from build123d import *

# Parameters (mm, degrees)
SKETCH1_W           = 200
SKETCH1_H           = 97
BOSS_EXTRUDE1_DEPTH = 20.75
SKETCH2_W           = 15
SKETCH2_H           = 96
CUT_EXTRUDE1_DEPTH  = 34
SKETCH3_W           = 6.3
SKETCH3_H           = 96
CUT_EXTRUDE2_DEPTH  = 40.5
SKETCH4_R           = 1.65
CUT_EXTRUDE3_DEPTH  = 2
SKETCH5_R           = 1.65
CUT_EXTRUDE4_DEPTH  = 42.5


with BuildPart() as part:
    # Sketch1 → Boss-Extrude1 (new body, symmetric)
    with BuildSketch(Plane(origin=(0, 0, 0), x_dir=(1, 0, 0), z_dir=(0, 1, 0))):
        Rectangle(SKETCH1_W, SKETCH1_H)
    extrude(amount=BOSS_EXTRUDE1_DEPTH, both=True)

    # Sketch2 → Cut-Extrude1 (cut)
    with BuildSketch(Plane(origin=(0, 20.75, 0), x_dir=(1, 0, 0), z_dir=(0, 1, 0))):
        with Locations((92.5, -0.5)):
            Rectangle(SKETCH2_W, SKETCH2_H)
    extrude(amount=-CUT_EXTRUDE1_DEPTH, mode=Mode.SUBTRACT)

    # Sketch3 → Cut-Extrude2 (cut)
    with BuildSketch(Plane(origin=(0, 20.75, 0), x_dir=(1, 0, 0), z_dir=(0, 1, 0))):
        with Locations((-96.85, -0.5)):
            Rectangle(SKETCH3_W, SKETCH3_H)
    extrude(amount=-CUT_EXTRUDE2_DEPTH, mode=Mode.SUBTRACT)

    # Sketch4 → Cut-Extrude3 (cut, through all)
    with BuildSketch(Plane.XY.offset(-47.5)):
        with Locations((94.25, 7.5)):
            Circle(SKETCH4_R)
        with BuildLine():
            Line((-96.35, 9.25), (-100, 9.25))
            Line((-100, 9.25), (-100, 5.95))
            Line((-100, 5.95), (-96.35, 5.95))
            ThreePointArc((-96.35, 5.95), (-94.7, 7.6), (-96.35, 9.25))
        make_face()
    extrude(amount=-CUT_EXTRUDE3_DEPTH, mode=Mode.SUBTRACT)

    # Sketch5 → Cut-Extrude4 (cut, through all)
    with BuildSketch(Plane.XZ.offset(20.75)):
        with Locations((97.25, -42.35)):
            Circle(SKETCH5_R)
    extrude(amount=-CUT_EXTRUDE4_DEPTH, mode=Mode.SUBTRACT)


solid = part.part
Read the model definition and answer for the solid it produces. Units are mm, in the model's axes. A direction names the side the tool comes from. Give positions to 0.01 mm unless a question says otherwise; leave off trailing zeros. Write each loop counter-clockwise with the first axis right and the second up, starting at its lowest first coordinate (ties: lowest second). Pieces come first, ordered by that corner, then holes. Notation, with made-up numbers: (54.5, -22.5) - (71.5, -22.5) arc R21 ccw to (71.5, 5.5) - close; hole circle Ø2 at (74, 1.5). An arc over 180 degrees is marked (long way). Use CSV: the item, a comma, the result in double quotes. Start each with the question number.
(1) Given P1, Ø4.5, axis at x = 93, z = 20, coming from the +Y side; P2, Ø10, axis at y = 1, z = 16, coming from the -X side; P3, Ø5, axis at x = -96.5, y = -3, coming from the +Z side, each flat-ended and moving along its own axis, determine where each tip first touches the part or whether it passes through.
(2) Find section B-B (y = -9). Give the vertices of the cut face in (x, z), plus the area to 3 significant figures.
(3) Consider line 1 along X through (y, z) = (-17, -42); line 2 along Y through (x, z) = (94.25, -47.75); line 3 along Z through (x, y) = (97, -18). Determine where each line is inside the solid, lowest interval first.
(4) For faces 1 (the flat face through (100, -17, 0)), 2 (the flat face through (-93.7, 1, 1)), 3 (the flat face through (85, 4, 1)), determine the directions among +Z, -Z, +X, -X, +Y, -Y from which every point of the face is accessible in a straight line to the end or side of a thin tool.
(5) Find section A-A (z = 6). Give the vertices of the cut face in (x, y), plus the area to 3 significant figures.
Findings below:
1,P1,"y = -13.25"
1,P2,"x = -93.7"
1,P3,"z = -47.5"
2,outline,"(-100, -48.5) - (100, -48.5) - (100, -47.5) - (85, -47.5) - (85, 48.5) - (-93.7, 48.5) - (-93.7, -47.5) - (-100, -47.5) - close"
2,area,"17,400 mm2"
3,line 1,"-93.7 to 95.64, 98.86 to 100"
3,line 2,"-20.75 to 5.85, 9.15 to 20.75"
3,line 3,"-48.5 to -43.98, -40.72 to 48.5"
4,face 1,"+Z, -Z, +X, +Y, -Y"
4,face 2,"+Z, -X, +Y"
4,face 3,"+Z, +X, +Y"
5,outline,"(-100, -20.75) - (100, -20.75) - (100, -13.25) - (85, -13.25) - (85, 20.75) - (-93.7, 20.75) - (-93.7, -19.75) - (-100, -19.75) - close"
5,area,"7,530 mm2"
